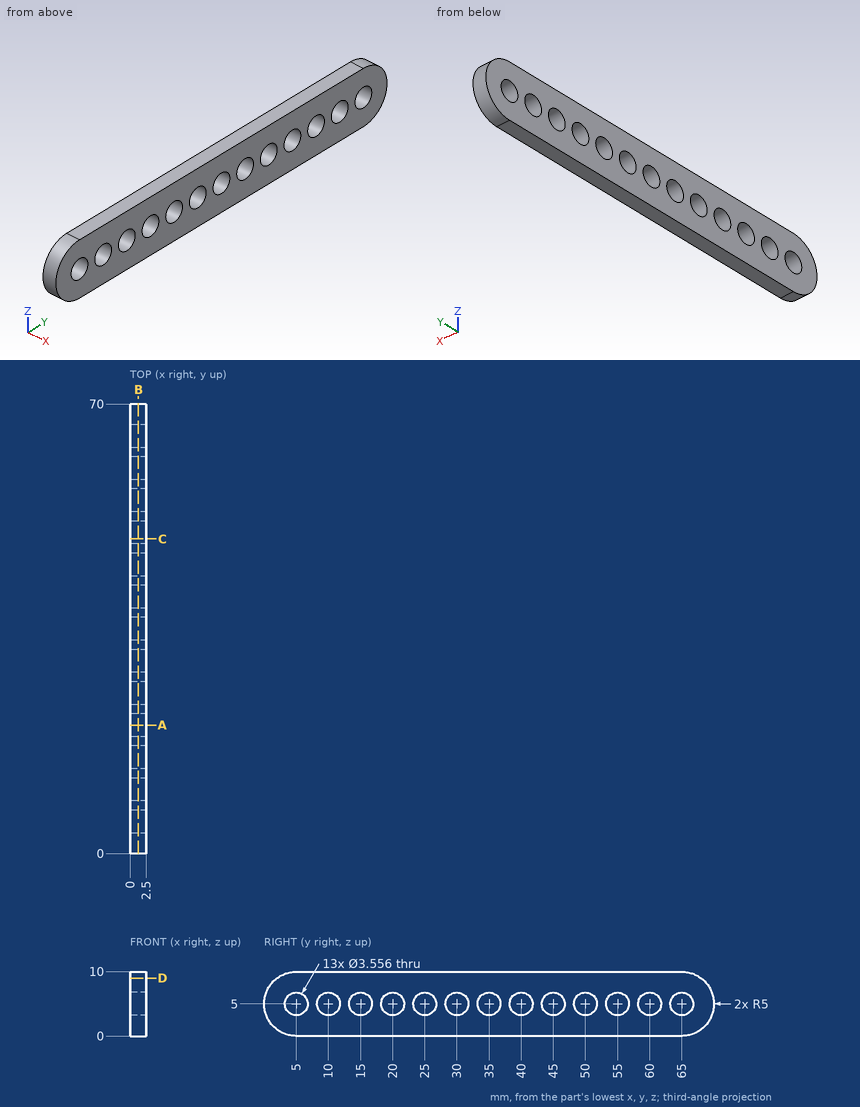
Job drawing, mm, ordinate dimensions from the low corner. One solid piece. Round coordinates to 2 decimals unless told otherwise and drop trailing zeros. Write each loop counter-clockwise with the first axis right and the second up, starting at its lowest first coordinate (ties: lowest second). Pieces come first, ordered by that corner, then holes. Notation, with made-up numbers: M 66,82.25 L 98,82.25 A25 ccw 98,104.25 Z; hole C -16.5,-13 d11. An arc over 180 degrees is marked long. Return JSON: item names as keys, results as strings. Group by question number.
(1) Saw through at C-C on y = 49. Write the cut outline in (x, z).
(2) Saw through at D-D on z = 9. Write the cut outline in (x, y).
(3) Pin check, flat tips, straight feed: pin 1 Ø2 at (y, z) = (25, 5) entering from -X (3 decimals); pin 2 Ø4.5 at (y, z) = (50, 5) entering from -X. Stop position of each tip, or through.
(4) Saw through at A-A on y = 20. Write the cut outline in (x, z), then the cut area to 3 significant figures.
(5) Drill centre lines: probe 1 along Z at (x, y) = (1.3, 65); probe 2 along Z at (x, y) = (1.3, 31); probe 3 along Y at (x, z) = (2.05, 8.5). Where is each one in solid material? Low to high.
(6) Saw through at B-B on x = 1.3. Count the separate pieces of the cut face and the enclosed holes in it, then the cut area to 3 significant figures.
Returned:
{
 "1": {"outline": "M 0,0 L 2.5,0 L 2.5,3.53 L 0,3.53 Z; M 0,6.47 L 2.5,6.47 L 2.5,10 L 0,10 Z"},
 "2": {"outline": "M 0,2 L 2.5,2 L 2.5,68 L 0,68 Z"},
 "3": {"pin 1": "through", "pin 2": "x = 0"},
 "4": {"outline": "M 0,0 L 2.5,0 L 2.5,3.22 L 0,3.22 Z; M 0,6.78 L 2.5,6.78 L 2.5,10 L 0,10 Z", "area": "16.1 mm²"},
 "5": {"probe 1": "0 to 3.22, 6.78 to 10", "probe 2": "0 to 3.53, 6.47 to 10", "probe 3": "1.43 to 68.57"},
 "6": {"separate pieces": "1", "enclosed holes": "13", "area": "549 mm²"}
}
